The figure shows three views and two pictorial views of one solid part (mm, origin at its lowest corner). Answer the questions. Round coordinates to 2 decimals unless told otherwise and drop trailing zeros. Order: outer loops, then holes, each group sorted by start corner. A loop starts at its lowest first (then second) coordinate and runs counter-clockwise, first axis right, second up. Notation, with made-up numbers: M 35,-8.5 L 89,-8.5 A27 cw 89,15.5 Z; hole C 88,46 d8. An arc over 180 degrees is marked long. Answer as CSV lines item,"result".
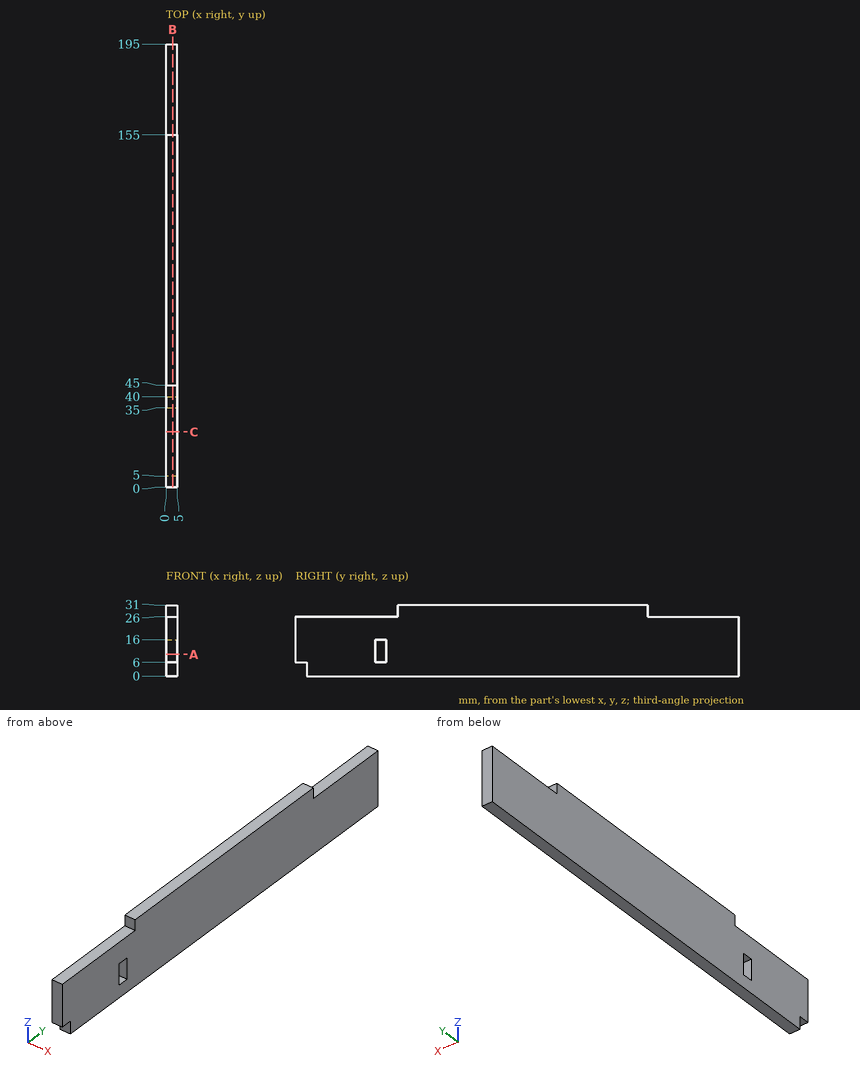
Item 1: A cutting plane is placed at A-A, the plane z = 9.5. Determine the outline of the cut face in (x, y), and give its area (3 significant figures).
Ans:
outline,"M 0,0 L 5,0 L 5,35 L 0,35 Z; M 0,40 L 5,40 L 5,195 L 0,195 Z"
area,"950 mm2"
Item 2: Flat-ended cylindrical pins translate along their axes: pin 1 (2 mm diameter, centred on x = 1.5, z = 22.5, fed in from -Y); pin 2 (2.5 mm diameter, centred on x = 2, z = 2, fed in from -Y); pin 3 (2.5 mm diameter, centred on x = 3, z = 28, fed in from -Y); pin 4 (1.5 mm diameter, centred on x = 1.5, y = 175.5, fed in from +Z). Find the tip coordinate at first contact, or state that the pin passes through.
Ans:
pin 1,"y = 0"
pin 2,"y = 5"
pin 3,"y = 45"
pin 4,"z = 26"
Item 3: A cutting plane is placed at B-B, the plane x = 2.9. Determine the outline of the cut face in (y, z), and give its area (3 significant figures).
Ans:
outline,"M 0,6 L 5,6 L 5,0 L 195,0 L 195,26 L 155,26 L 155,31 L 45,31 L 45,26 L 0,26 Z; hole M 35,6 L 40,6 L 40,16 L 35,16 Z"
area,"5,540 mm2"
Item 4: A cutting plane is placed at C-C, the plane y = 24.5. Determine the outline of the cut face in (x, z), and give its area (3 significant figures).
Ans:
outline,"M 0,0 L 5,0 L 5,26 L 0,26 Z"
area,"130 mm2"
Item 5: Find the intervals of material crossed by probe 1 along Y at (x, z) = (4.25, 8); probe 2 along Z at (x, y) = (3.2, 157); probe 3 along Y at (x, z) = (4.4, 28.5), in increasing order. Write a range as [from, to].
Ans:
probe 1,"[0, 35], [40, 195]"
probe 2,"[0, 26]"
probe 3,"[45, 155]"
